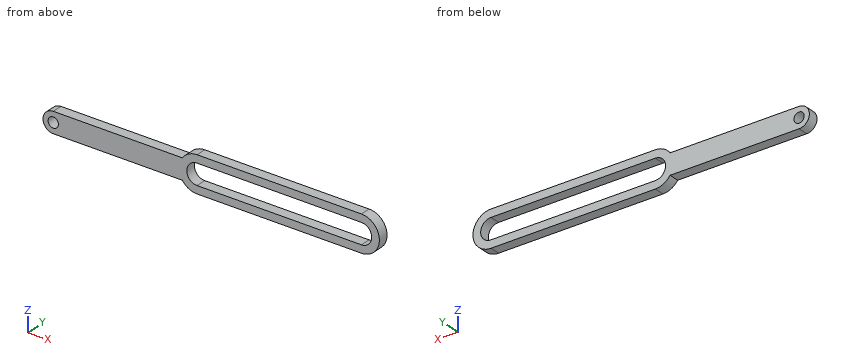
```python
from build123d import *

# Parameters (mm, degrees)
SKETCH_1_R      = 1
EXTRUDE_1_DEPTH = 2


with BuildPart() as part:
    # 草图1 → 凸台-拉伸1 (new body)
    with BuildSketch(Plane(origin=(0, 0, 0), x_dir=(1, 0, 0), z_dir=(0, 1, 0))):
        with BuildLine():
            Line((-30, 2), (-4.872281323, 2))
            ThreePointArc((-4.872281323, 2), (-3.620185175, 3.102418411), (-2, 3.5))
            Line((-2, 3.5), (30, 3.5))
            ThreePointArc((30, 3.5), (33.5, 0), (30, -3.5))
            Line((30, -3.5), (-2, -3.5))
            ThreePointArc((-2, -3.5), (-3.620185175, -3.102418411), (-4.872281323, -2))
            Line((-4.872281323, -2), (-30, -2))
            ThreePointArc((-30, -2), (-32, 0), (-30, 2))
        make_face()
        with Locations(Location((-30, 0, 0), (0, 0, 270))):
            Circle(SKETCH_1_R, mode=Mode.SUBTRACT)
        with BuildLine():
            Line((-2, 2), (30, 2))
            ThreePointArc((30, 2), (32, 0), (30, -2))
            Line((30, -2), (-2, -2))
            ThreePointArc((-2, -2), (-4, 0), (-2, 2))
        make_face(mode=Mode.SUBTRACT)
    extrude(amount=EXTRUDE_1_DEPTH)


solid = part.part
```
The listing builds one solid part. Answer for the finished solid, in the listing's coordinates (mm). Give positions to 0.01 mm unless a question says otherwise; leave off trailing zeros. Order: outer loops, then holes, each group sorted by start corner. A loop starts at its lowest first (then second) coordinate and runs counter-clockwise, first axis right, second up. Notation, with made-up numbers: M 72,36 L 95,36 A20 ccw 95,68 Z; hole C 82,-29 d4. An arc over 180 degrees is marked long. Put each result on its own line as item: value. Start each with the question number.
Item 1: The part is cut by section B-B, the plane x = 7.5. Determine the outline of the cut face in (y, z), and give its area (3 significant figures).
Item 2: The part is cut by section C-C, the plane y = 1.7. Determine the outline of the cut face in (x, z).
Item 3: Find the intervals of material crossed by line 1 along X through (y, z) = (0.6, 0); line 2 along Z through (x, y) = (25, 1.9); line 3 along X through (y, z) = (0.7, -0.75), in increasing order.
Item 4: The part is cut by section A-A, the plane z = 0. Determine the outline of the cut face in (x, y), and give its area (3 significant figures).
Item 5: The part is cut by section D-D, the plane x = -12. Determine the outline of the cut face in (y, z), and give its area (3 significant figures).
Item 6: Flat-ended cylindrical pins translate along their axes: P1, Ø0.6, axis at x = -13, y = 0.5, coming from the +Z side; P2, Ø0.6, axis at x = -15, y = 1.5, coming from the -Z side. Find the tip coordinate at first contact, or state that the pin passes through.
Answer key:
1. outline: M 0,-3.5 L 2,-3.5 L 2,-2 L 0,-2 Z; M 0,2 L 2,2 L 2,3.5 L 0,3.5 Z
1. area: 6.00 mm²
2. outline: M -30,-2 L -4.87,-2 A3.5 ccw -2,-3.5 L 30,-3.5 A3.5 ccw 30,3.5 L -2,3.5 A3.5 ccw -4.87,2 L -30,2 A2 ccw Z; hole C -30,0 d2; hole M -2,-2 L 30,-2 A2 ccw 30,2 L -2,2 A2 ccw Z
3. line 1: x = -32 to -31, -29 to -4, 32 to 33.5
3. line 2: z = -3.5 to -2, 2 to 3.5
3. line 3: x = -31.85 to -30.66, -29.34 to -3.85, 31.85 to 33.42
4. outline: M -32,0 L -31,0 L -31,2 L -32,2 Z; M -29,0 L -4,0 L -4,2 L -29,2 Z; M 32,0 L 33.5,0 L 33.5,2 L 32,2 Z
4. area: 55.0 mm²
5. outline: M 0,-2 L 2,-2 L 2,2 L 0,2 Z
5. area: 8.00 mm²
6. P1: stops at z = 2
6. P2: stops at z = -2
